Can you work these out from the model? Positions are in its coordinate system, mm. Give positions to 0.01 mm unless a question says otherwise; leave off trailing zeros. Loops run counter-clockwise (first coordinate to the right, second up) from the corner with the lowest first, then second, coordinate; pieces in that order, holes last. Notation, with made-up numbers: (50.5, 1.25) -> (106.5, 1.25) arc R24 cw to (106.5, 30.25) -> close; hole circle Ø2 at (-17.75, 1). An arc over 180 degrees is marked (long way). One line per question, with ' | ' between items.
from build123d import *

# Parameters (mm, degrees)
F1_DEPTH = 240
F2_DEPTH = 2
F4_DEPTH = 2


with BuildPart() as f1:
    # F0 (on Front) → F1 (new body)
    with BuildSketch(Plane.XZ):
        with BuildLine():
            ThreePointArc((-6, -8.919781), (-5.280189, -9.363872), (-4.527693, -9.75))
            Line((-4.527693, -9.75), (0, -9.75))
            ThreePointArc((0, -9.75), (-8.415191, -4.924131), (-8.5, 4.776243))
            Line((-8.5, 4.776243), (-9.934369, 4.107408))
            ThreePointArc((-9.934369, 4.107408), (-10.290916, -3.107982), (-6, -8.919781))
        make_face()
        with BuildLine():
            ThreePointArc((8.5, 4.776243), (8.415191, -4.924131), (0, -9.75))
            Line((0, -9.75), (4.527693, -9.75))
            ThreePointArc((4.527693, -9.75), (5.280189, -9.363872), (6, -8.919781))
            ThreePointArc((6, -8.919781), (10.290916, -3.107982), (9.934369, 4.107408))
            Line((9.934369, 4.107408), (8.5, 4.776243))
        make_face()
        with BuildLine():
            Line((0, -9.75), (-4.527693, -9.75))
            ThreePointArc((-4.527693, -9.75), (-5.280189, -9.363872), (-6, -8.919781))
            Line((-6, -8.919781), (-6, -9.75))
            Line((-6, -9.75), (-6, -10.15))
            Line((-6, -10.15), (6, -10.15))
            Line((6, -10.15), (6, -9.75))
            Line((6, -9.75), (6, -8.919781))
            ThreePointArc((6, -8.919781), (5.280189, -9.363872), (4.527693, -9.75))
            Line((4.527693, -9.75), (0, -9.75))
        make_face()
    extrude(amount=F1_DEPTH)

    # F0 (on Front) → F2 (join)
    with BuildSketch(Plane.XZ):
        with BuildLine():
            ThreePointArc((-8.5, 4.776243), (-8.415191, -4.924131), (0, -9.75))
            ThreePointArc((0, -9.75), (8.415191, -4.924131), (8.5, 4.776243))
            Line((8.5, 4.776243), (-8.5, 4.776243))
        make_face()
    extrude(amount=F2_DEPTH)

    # F3 (on face) → F4 (join)
    with BuildSketch(Plane.XZ.offset(240)):
        with BuildLine():
            Line((8.5, 4.776243), (-8.5, 4.776243))
            ThreePointArc((-8.5, 4.776243), (0, -9.75), (8.5, 4.776243))
        make_face()
    extrude(amount=-F4_DEPTH)


solid = f1.part
Q1. If I drill on probe 1 along Y at (x, z) = (3, -9); probe 2 along X at (y, z) = (-132.5, 0.5); probe 3 along X at (y, z) = (-163.5, -5), over which ranges is the centre line in solid material (lowest first)? Write a range as from..to.
Entries:
probe 1: -240..-238, -2..0 | probe 2: -10.74..-9.74, 9.74..10.74 | probe 3: -9.52..-8.37, 8.37..9.52
Q2. If we mould it in two halves opening along Y, with no side actions, what happens to faces 1 (the face through (0, -240, -3)), 2 (the face through (0, -238, -1)), 3 (the face through (10.26, -118.32, -3.21)), 4 (the face through (0, -2, -1))? For each: pulls with the +Y half, pulls with the -Y half, needs draft (parallel to the pull), parting line crosses it, or undercut.
Entries:
face 1: pulls with the -Y half | face 2: undercut | face 3: needs draft | face 4: undercut
Q3. If we section it at A-A (y = -184.5): Write out the boundary of the cut face in (x, z).
Entries:
outline: (-9.93, 4.11) arc R10.75 ccw to (-6, -8.92) -> (-6, -10.15) -> (6, -10.15) -> (6, -8.92) arc R10.75 ccw to (9.93, 4.11) -> (8.5, 4.78) arc R9.75 cw to (0, -9.75) arc R9.75 cw to (-8.5, 4.78) -> close
Q4. For pin 1 Ø3 at (x, y) = (-5, -105.5) entering from +Z; pin 2 Ø5 at (x, y) = (6.5, -27) entering from +Z; pin 3 Ø1 at (y, z) = (-137, -9.5) entering from -X, each with a flat end and sliding along its axis, tell me the tip position at first contact or that it passes through.
Entries:
pin 1: z = -7.27 | pin 2: z = 4.78 | pin 3: x = -6
Q5. If we section it at B-B (z = 1): Write out the boundary of the cut face in (x, y), plus the area to 3 significant figures.
Entries:
outline: (-10.7, -240) -> (10.7, -240) -> (10.7, 0) -> (-10.7, 0) -> close; hole (-9.7, -238) -> (9.7, -238) -> (9.7, -2) -> (-9.7, -2) -> close | area: 560 mm²
